from build123d import *

# Parameters (mm, degrees)
F1_DEPTH  = 76.2
F2_R      = 9.525
F4_W      = 19.05
F4_H      = 19.05
F5_DEPTH  = 3.175
F6_W      = 2.54
F6_H      = 44.45
F6_W_2    = 44.45
F6_H_2    = 2.54
F7_DEPTH  = 3.175
F8_R      = 5.08
F9_W      = 24.864539
F9_H      = 7.45066
F9_W_2    = 9.066464
F9_H_2    = 23.017317
F10_DEPTH = 1.5875


with BuildPart() as f1:
    # F0 (on Top) → F1 (new body)
    with BuildSketch(Plane.XY):
        Polygon((-12.7, 0), (0, 0), (0, 59.266667), (-12.7, 59.266667), (-12.7, 12.7), (-59.266667, 12.7), (-59.266667, 0), align=None)
    extrude(amount=F1_DEPTH)

    # F2
    f2_edges = [f1.edges().sort_by_distance(p)[0] for p in [
        (-12.7, 12.7, 38.1),
        (0, 0, 38.1),
    ]]
    fillet(f2_edges, radius=F2_R)

    # F4 (on offset) → F5 (cut)
    with BuildSketch(Plane.XY.offset(76.2)):
        with Locations((-9.525, 9.525)):
            Rectangle(F4_W, F4_H)
    extrude(amount=-F5_DEPTH, mode=Mode.SUBTRACT)

    # F6 (on offset) → F7 (cut)
    with BuildSketch(Plane.XY.offset(76.2)):
        with Locations((-7.62, 40.052507)):
            Rectangle(F6_W, F6_H)
        with Locations((-39.902898, 7.62)):
            Rectangle(F6_W_2, F6_H_2)
    extrude(amount=-F7_DEPTH, mode=Mode.SUBTRACT)

    # F8
    f8_edges = [f1.edges().sort_by_distance(p)[0] for p in [
        (-59.266667, 0, 38.1),
        (-59.266667, 12.7, 38.1),
        (-12.7, 59.266667, 38.1),
        (0, 59.266667, 38.1),
    ]]
    fillet(f8_edges, radius=F8_R)

    # F9 (on offset) → F10 (cut)
    with BuildSketch(Plane.XY.offset(76.2)):
        with Locations((-48.689407, 11.571373)):
            Rectangle(F9_W, F9_H)
        with Locations((-11.794715, 50.10781)):
            Rectangle(F9_W_2, F9_H_2)
    extrude(amount=-F10_DEPTH, mode=Mode.SUBTRACT)


solid = f1.part
Geometry: final body of the model. Coordinates: model frame, mm. A direction names the side the tool comes from. Coordinates: 2 decimals unless noted, no trailing zeros. Write each loop counter-clockwise with the first axis right and the second up, starting at its lowest first coordinate (ties: lowest second). Pieces come first, ordered by that corner, then holes. Notation, with made-up numbers: (-32, 40.5) - (12, 40.5) arc R24 ccw to (12, 71.5) - close; hole circle Ø3 at (59.25, 79.5). An arc over 180 degrees is marked (long way). Return JSON: item names as keys, results as strings.
Item 1: Section query A-A (x = -33). Output: boundary loops of the cut face in (y, z) (3 decimals).
Completed:
{"outline": "(0, 0) - (12.7, 0) - (12.7, 76.2) - (8.89, 76.2) - (8.89, 73.025) - (6.35, 73.025) - (6.35, 76.2) - (0, 76.2) - close"}
Item 2: Line query: L1, parallel to Y at x = -46, z = 55; L2, parallel to X at y = 45.5, z = 40; L3, parallel to Z at x = -12, y = 55. Output: solid intervals per line, ascending.
Completed:
{"L1": "y = 0 to 12.7", "L2": "x = -12.7 to 0", "L3": "z = 0 to 74.61"}
Item 3: Pin query (flat end, axial travel): pin 1 Ø0.8 at (y, z) = (10.5, 75.5) entering from -X; pin 2 Ø10 at (y, z) = (15, 65.5) entering from -X; pin 3 Ø1.6 at (y, z) = (11.5, 74) entering from +X. Return the tip coordinate at first contact, or that it passes through.
Completed:
{"pin 1": "stops at x = -36.26", "pin 2": "stops at x = -58.67", "pin 3": "stops at x = -19.05"}
Item 4: Section query C-C (z = 28). Output: boundary loops of the cut face in (x, y) (3 decimals), and give its area (3 significant figures).
Completed:
{"outline": "(-59.267, 5.08) arc R5.08 ccw to (-54.187, 0) - (-9.525, 0) arc R9.525 ccw to (0, 9.525) - (0, 54.187) arc R5.08 ccw to (-5.08, 59.267) - (-7.62, 59.267) arc R5.08 ccw to (-12.7, 54.187) - (-12.7, 22.225) arc R9.525 cw to (-22.225, 12.7) - (-54.187, 12.7) arc R5.08 ccw to (-59.267, 7.62) - close", "area": "1,320 mm2"}
Item 5: Pull-direction query (X, two-part tool) for faces 1 (the face through (-59.267, 6, 38)), 2 (the face through (-39, 3, 76.2)), 3 (the face through (-6.35, 39, 75)); classes: +X half, -X half, draft (parallel to the pull), parting line (faces both ways), or undercut.
Completed:
{"face 1": "-X half", "face 2": "draft", "face 3": "undercut"}
Item 6: Section query D-D (x = -15). Output: boundary loops of the cut face in (y, z) (3 decimals).
Completed:
{"outline": "(0, 0) - (16.018, 0) - (16.018, 73.025) - (0, 73.025) - close"}
Item 7: Reachability of faces 4 (the face through (-35, 8.89, 74)), 5 (the face through (-38, 12.7, 38)), 6 (the face through (-11, 49, 74.612)), 7 (the face through (-19.05, 3, 75)), 8 (the face through (-3, 19.05, 75)) from +Z, -Z, +X, -X, +Y, -Y: full face, straight path, thin tool, end or side. Return the list, or none.
Completed:
{"face 4": "+Z, +X, -X", "face 5": "+Z, -Z, -X, +Y", "face 6": "+Z, -X, +Y", "face 7": "+Z, +X, +Y, -Y", "face 8": "+Z, +X, -X, -Y"}
